from build123d import *

# Parameters (mm, degrees)
SKETCH1_W          = 50
SKETCH1_H          = 20
EXTRUDE1_DEPTH     = 10
SKETCH2_W          = 6
SKETCH2_H          = 16
CUT_EXTRUDE1_DEPTH = 60
CUT_EXTRUDE2_DEPTH = 30


with BuildPart() as part:
    # Sketch1 → Extrude1 (new body)
    with BuildSketch(Plane.XY):
        with Locations((-71.138674094, 124.333988555)):
            Rectangle(SKETCH1_W, SKETCH1_H)
    extrude(amount=EXTRUDE1_DEPTH)

    # Sketch2 → Cut-Extrude1 (cut)
    with BuildSketch(Plane.ZY.offset(96.138674094)):
        with Locations((5, 124.333988555)):
            Rectangle(SKETCH2_W, SKETCH2_H)
    extrude(amount=-CUT_EXTRUDE1_DEPTH, mode=Mode.SUBTRACT)

    # Sketch3 → Cut-Extrude2 (cut)
    with BuildSketch(Plane.XY.offset(10)):
        with BuildLine():
            ThreePointArc((-56.138674094, 127.833988555), (-58.638674094, 125.333988555), (-56.138674094, 122.833988555))
            ThreePointArc((-56.138674094, 122.833988555), (-53.638674094, 125.333988555), (-56.138674094, 127.833988555))
        make_face()
        with BuildLine():
            ThreePointArc((-86.138674094, 127.833988555), (-88.638674094, 125.333988555), (-86.138674094, 122.833988555))
            ThreePointArc((-86.138674094, 122.833988555), (-83.638674094, 125.333988555), (-86.138674094, 127.833988555))
        make_face()
    extrude(amount=-CUT_EXTRUDE2_DEPTH, mode=Mode.SUBTRACT)


solid = part.part
Could you check a few things on this model? Use its own coordinates, in mm. A direction names the side the tool comes from. Coordinates: 2 decimals unless noted, no trailing zeros. Write each loop counter-clockwise with the first axis right and the second up, starting at its lowest first coordinate (ties: lowest second). Pieces come first, ordered by that corner, then holes. Notation, with made-up numbers: M 73.25,50 L 128.25,50 A17 cw 128.25,60 Z; hole C 51.25,-19.5 d1. An arc over 180 degrees is marked long. One line per question, with ' | ' between items.
1) Imagine slicing it at C-C, the plane x = -61.5. Write out the boundary of the cut face in (y, z).
Checks:
outline: M 114.33,0 L 134.33,0 L 134.33,10 L 114.33,10 Z; hole M 116.33,2 L 132.33,2 L 132.33,8 L 116.33,8 Z
2) I need wall thicknesses on probe 1 along Z at (x, y) = (-71.5, 117.75); probe 2 along Y at (x, z) = (-69, 2.5). Which ranges of each line are inside material? Lowest first, please. Write a range as [from, to].
Checks:
probe 1: [0, 2], [8, 10] | probe 2: [114.33, 116.33], [132.33, 134.33]
3) Imagine slicing it at B-B, the plane z = 6.5. Write out the boundary of the cut face in (x, y), and give its area (3 significant figures).
Checks:
outline: M -96.14,114.33 L -46.14,114.33 L -46.14,116.33 L -96.14,116.33 Z; M -96.14,132.33 L -46.14,132.33 L -46.14,134.33 L -96.14,134.33 Z | area: 200 mm²
4) Imagine slicing it at A-A, the plane y = 121.25. Write out the boundary of the cut face in (x, z), and give its area (3 significant figures).
Checks:
outline: M -96.14,0 L -46.14,0 L -46.14,2 L -96.14,2 Z; M -96.14,8 L -46.14,8 L -46.14,10 L -96.14,10 Z | area: 200 mm²
5) Imagine slicing it at D-D, the plane y = 124.75. Write out the boundary of the cut face in (x, z), and give its area (3 significant figures).
Checks:
outline: M -96.14,0 L -88.57,0 L -88.57,2 L -96.14,2 Z; M -96.14,8 L -88.57,8 L -88.57,10 L -96.14,10 Z; M -83.71,0 L -58.57,0 L -58.57,2 L -83.71,2 Z; M -83.71,8 L -58.57,8 L -58.57,10 L -83.71,10 Z; M -53.71,0 L -46.14,0 L -46.14,2 L -53.71,2 Z; M -53.71,8 L -46.14,8 L -46.14,10 L -53.71,10 Z | area: 161 mm²
6) For faces 1 (the face through (-83.66, 125.66, 9.01)), 2 (the face through (-71, 124, 8)), which set-ups out of +Z, -Z, +X, -X, +Y, -Y let a thin tool reach every point of the face, with its end or its side?
Checks:
face 1: +Z, -Z | face 2: +X, -X
7) If we mould it in two halves opening along Z, with no side actions, what happens to faces 3 (the face through (-71, 124, 0)), 4 (the face through (-71, 116.334, 5)), 5 (the face through (-46.139, 124.2, 1.6))? For each: released by +Z, released by -Z, zero draft, split by the parting line, or undercut.
Checks:
face 3: released by -Z | face 4: undercut | face 5: zero draft
